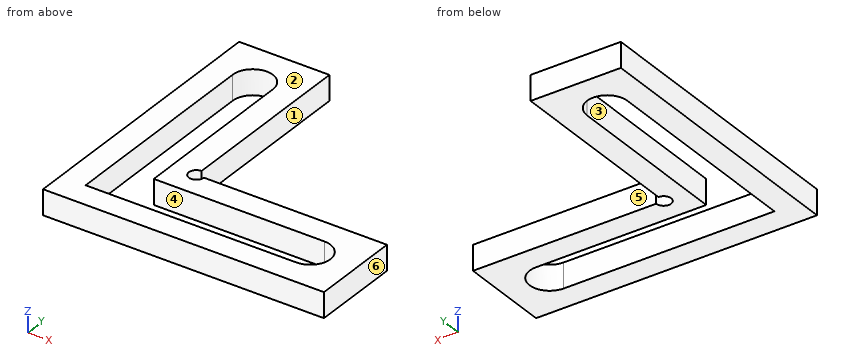
Autodesk Inventor part; units mm, degrees
ref_plane "YZ Plane" through (0, 0, 0) normal (1, 0, 0) x (0, 1, 0)
ref_plane "XZ Plane" through (0, 0, 0) normal (0, 1, 0) x (-1, 0, 0)
ref_plane "XY Plane" through (0, 0, 0) normal (0, 0, 1) x (1, 0, 0)
sketch "Sketch1" plane through (0, 0, 0) normal (0, 0, 1) x (1, 0, 0)
  line L0 (0, 0) -> (0, 50)
  line L1 (0, 50) -> (12, 50)
  line L2 (12, 50) -> (12, 12)
  line L3 (12, 12) -> (50, 12)
  line L4 (50, 12) -> (50, 0)
  line L5 (50, 0) -> (0, 0)
  dimension "d0" = 50
  dimension "d1" = 12
  dimension "d2" = 38
  dimension "d3" = 38
extrude "Extrusion1" add sketch "Sketch1" along normal blind 5
sketch "Sketch2" plane through (0, 0, 5) normal (0, 0, 1) x (1, 0, 0)
  line L0 (10, 44) -> (10, 2)
  line L1 (10, 2) -> (2, 2)
  line L2 (2, 2) -> (2, 44)
  line L3 (12, 12) -> (12, 50)
  line L4 (12, 50) -> (0, 50)
  arc A0 (10, 44) -> (2, 44) centre (6, 44) ccw
  line L5 (0, 0) -> (50, 0)
  line L6 (2, 2) -> (44, 2)
  line L7 (44, 10) -> (2, 10)
  line L8 (2, 10) -> (2, 2)
  arc A1 (44, 2) -> (44, 10) centre (44, 6) ccw
  line L9 (50, 0) -> (50, 12)
  line L10 (50, 12) -> (12, 12)
  point P0 (10, 2)
  point P1 (10, 10)
  dimension "d6" = 8
  dimension "d7" = 2
  dimension "d9" = 4
  dimension "d10" = 6
  dimension "d11" = 2
  dimension "d12" = 8
  dimension "d13" = 6
  dimension "d14" = 2
  dimension "d15" = 4
extrude "Extrusion2" cut sketch "Sketch2" against normal through all
sketch "Sketch3" plane through (0, 0, 5) normal (0, 0, 1) x (1, 0, 0)
  line L0 (15, 15) -> (15, 50)
  line L1 (-3, 50) -> (-3, 0)
  line L2 (15, 15) -> (53, 15)
  line L3 (50, -3) -> (-3, -3)
  line L4 (-3, -3) -> (-3, 16.0843)
  line L5 (0, 50) -> (0, 0)
  line L6 (12, 12) -> (12, 50)
  line L7 (50, 12) -> (12, 12)
  line L8 (0, 0) -> (50, 0)
  line L9 (15, 50) -> (15, 53)
  line L10 (15, 53) -> (-3, 53)
  line L11 (-3, 53) -> (-3, 50)
  line L12 (50, -3) -> (53, -3)
  line L13 (53, -3) -> (53, 15)
  line L14 (12, 50) -> (0, 50)
  line L15 (50, 0) -> (50, 12)
  dimension "d18" = 3
  dimension "d19" = 3
  dimension "d20" = 3
  dimension "d21" = 3
  dimension "d24" = 3
  dimension "d25" = 3
extrude "Extrusion3" add sketch "Sketch3" against normal blind 5
sketch "Sketch4" plane through (0, 0, 5) normal (0, 0, 1) x (1, 0, 0)
  line L0 (53, 15) -> (15, 15)
  circle A0 centre (15, 15) radius 1.5
  point P0 (0, 0)
  dimension "d28" = 3
extrude "Extrusion4" cut sketch "Sketch4" against normal blind 5
properties part number "Kabelhalterung_V1"
The model under review builds one solid part; all positions refer to its coordinate system, in mm. Face numbers are marked on the shaded views. A direction names the side the tool comes from. Round coordinates to 2 decimals unless told otherwise and drop trailing zeros. Loops run counter-clockwise (first coordinate to the right, second up) from the corner with the lowest first, then second, coordinate; pieces in that order, holes last. Notation, with made-up numbers: M -30.5,-30 L 0.5,-30 A33 ccw 0.5,-1 Z; hole C 86.25,-17.75 d4. An arc over 180 degrees is marked long. Write item = value, one per line.
Item 1: Take a section at A-A on x = 36. Write out the cut boundary in (y, z), then the cut area to 3 significant figures.
Return value:
outline = M -3,0 L 2,0 L 2,5 L -3,5 Z; M 10,0 L 15,0 L 15,5 L 10,5 Z
area = 50.0 mm2
Item 2: Take a section at C-C on y = 6. Write out the cut boundary in (x, z), then the cut area to 3 significant figures.
Return value:
outline = M -3,0 L 2,0 L 2,5 L -3,5 Z; M 48,0 L 53,0 L 53,5 L 48,5 Z
area = 50.0 mm2
Item 3: The part is to be moulded in two halves that separate along Y. For the marked faces 4, 5 and 6, say which applies: released by +Y, released by -Y, zero draft, split by the parting line, or undercut.
Return value:
face_4 = undercut
face_5 = released by +Y
face_6 = zero draft
Item 4: Take a section at B-B on z = 0.8. Write out the cut boundary in (x, y).
Return value:
outline = M -3,-3 L 53,-3 L 53,15 L 16.5,15 A1.5 cw long 15,16.5 L 15,53 L -3,53 Z; hole M 2,2 L 44,2 A4 ccw 44,10 L 10,10 L 10,44 A4 ccw 2,44 Z
Item 5: Insertion check: P1, Ø1.5, axis at y = 17.5, z = 3.5, coming from the +X side; P2, Ø5, axis at x = 15, y = 15, coming from the -Z side; P3, Ø2.5, axis at x = 21.5, z = 2, coming from the +Y side. Each pin has a flat end and moves straight along its axis. Give the tip position at first contact, or say it passes through.
Return value:
P1 = 15
P2 = 0
P3 = 15
Item 6: For line 1 (X direction, y = 6, z = 1.55); line 2 (X direction, y = 22, z = 2.55), list the stretches that pass through material, from the lowest coordinate up. Write a range as [from, to].
Return value:
line_1 = [-3, 2], [48, 53]
line_2 = [-3, 2], [10, 15]
Item 7: Machinability: for the marked faces 1, 2 and 3, which of the approach directions +Z, -Z, +X, -X, +Y, -Y give a long, thin tool a straight path to every point of the face, cutting with its end or side? Answer none if there is none.
Return value:
face_1 = +Z, -Z, +X, +Y
face_2 = +Z, +X, -X, +Y, -Y
face_3 = +Z, -Z
